```python
from build123d import *

# Parameters (mm, degrees)
SKETCH_W        = 60
SKETCH_H        = 30
SKETCH_R        = 2.25
SKETCH_R_2      = 2.2
PAD_DEPTH       = 2.8
SKETCH001_W     = 75
SKETCH001_H     = 45
POCKET_DEPTH    = 2.801
SKETCH002_R     = 2.2
PAD001_DEPTH    = 24
SKETCH003_R     = 8.1
POCKET001_DEPTH = 3.8
CHAMFER_SIZE    = 2
FILLET_R        = 2
FILLET001_R     = 2


with BuildPart() as part:
    # Sketch → Pad (new body)
    with BuildSketch(Plane.XY):
        Rectangle(SKETCH_W, SKETCH_H)
        with Locations((25, 0)):
            Circle(SKETCH_R, mode=Mode.SUBTRACT)
        with Locations((-25, 0)):
            Circle(SKETCH_R, mode=Mode.SUBTRACT)
        Circle(SKETCH_R_2, mode=Mode.SUBTRACT)
    extrude(amount=PAD_DEPTH)

    # Sketch001 → Pocket (cut, through all)
    with BuildSketch(Plane.XY.offset(2.8)):
        Rectangle(SKETCH001_W, SKETCH001_H)
        with BuildLine():
            ThreePointArc((-27, 9.5), (-24.525126, 10.525126), (-23.5, 13))
            Line((-23.5, 13), (-23.5, 18))
            Line((-23.5, 18), (-3.5, 18))
            Line((-3.5, 18), (-3.5, 13))
            ThreePointArc((-3.5, 13), (0, 9.5), (3.5, 13))
            Line((3.5, 13), (3.5, 18))
            Line((3.5, 18), (23.5, 18))
            Line((23.5, 18), (23.5, 13))
            ThreePointArc((23.5, 13), (24.525126, 10.525126), (27, 9.5))
            Line((27, 9.5), (32, 9.5))
            Line((32, 9.5), (32, -9.5))
            Line((32, -9.5), (27, -9.5))
            ThreePointArc((27, -9.5), (24.525128, -10.525124), (23.5, -12.999994))
            Line((23.5, -12.999994), (23.5, -17.999994))
            Line((23.5, -17.999994), (3.5, -17.999994))
            Line((3.5, -12.999994), (3.5, -17.999994))
            ThreePointArc((3.5, -12.999994), (-4e-06, -9.5), (-3.5, -13.000002))
            Line((-3.5, -13.000002), (-3.5, -18.000002))
            Line((-23.499999, -18.000002), (-3.5, -18.000002))
            Line((-23.499999, -18.000002), (-23.499999, -13.000002))
            ThreePointArc((-23.499999, -13.000002), (-24.525131, -10.525138), (-27, -9.500018))
            Line((-27, -9.500018), (-32, -9.500018))
            Line((-32, -9.500018), (-32, 9.5))
            Line((-32, 9.5), (-27, 9.5))
        make_face(mode=Mode.SUBTRACT)
    extrude(amount=-POCKET_DEPTH, mode=Mode.SUBTRACT)

    # Sketch002 → Pad001 (new body)
    with BuildSketch(Plane.XY.offset(2.8)):
        with BuildLine():
            Line((-10, -10), (-10, 10))
            Line((-10, 10), (-1.802776, 10))
            ThreePointArc((-1.802776, 10), (0, 9.5), (1.802776, 10))
            Line((1.802776, 10), (10, 10))
            Line((10, 10), (10, -10))
            Line((1.802776, -10), (10, -10))
            ThreePointArc((1.802776, -10), (0, -9.5), (-1.802776, -10))
            Line((-1.802776, -10), (-10, -10))
        make_face()
        Circle(SKETCH002_R, mode=Mode.SUBTRACT)
    extrude(amount=PAD001_DEPTH)

    # Sketch003 → Pocket001 (cut)
    with BuildSketch(Plane.XY.offset(26.8)):
        Circle(SKETCH003_R)
    extrude(amount=-POCKET001_DEPTH, mode=Mode.SUBTRACT)

    # Chamfer
    chamfer_edges = [part.edges().sort_by_distance(p)[0] for p in [
        (-10, -10, 14.8),
        (10, -10, 14.8),
        (-10, 10, 14.8),
        (10, 10, 14.8),
    ]]
    chamfer(chamfer_edges, length=CHAMFER_SIZE)

    # Fillet
    fillet_edges = [part.edges().sort_by_distance(p)[0] for p in [
        (-10, 0, 2.8),
    ]]
    fillet(fillet_edges, radius=FILLET_R)

    # Fillet001
    fillet001_edges = [part.edges().sort_by_distance(p)[0] for p in [
        (10, 0, 2.8),
    ]]
    fillet(fillet001_edges, radius=FILLET001_R)


solid = part.part
```
Verification items for the finished model (mm, model axes). A direction names the side the tool comes from. Give positions to 0.01 mm unless a question says otherwise; leave off trailing zeros. Order: outer loops, then holes, each group sorted by start corner. A loop starts at its lowest first (then second) coordinate and runs counter-clockwise, first axis right, second up. Notation, with made-up numbers: M 8,75.5 L 62,75.5 A15 ccw 62,96.5 Z; hole C -11.75,76.5 d5. An arc over 180 degrees is marked long. Answer in a Markdown table with one row per item. Add a question column.
Item 1: Section check B-B, the plane y = 0. Enter the section's corners in (x, z), and give its area (3 significant figures).
Item 2: Tool access check on faces 4 (the flat face through (-28, -9.5, 1)), 5 (the flat face through (-29, 9.5, 1)), 6 (the flat face through (29, -9.5, 1)). Record the directions out of +Z, -Z, +X, -X, +Y, -Y that give a thin tool (end or side, any length) a straight path to the whole face; none if there is none.
Item 3: Section check D-D, the plane x = 9. Enter the section's corners in (y, z), and give its area (3 significant figures).
Item 4: Scan lines: probe 1 along Y at (x, z) = (0, 15); probe 2 along Y at (x, z) = (0, 24); probe 3 along Z at (x, y) = (14.5, -10). Record each from-to range of solid material in increasing order. Write a range as from..to.
Item 5: Section check C-C, the plane z = 15. Enter the section's corners in (x, y), and give its area (3 significant figures).
Item 6: Section check A-A, the plane x = 0. Enter the section's corners in (y, z).
Item 7: Gauge pin test, flat ends, axial feed: pin 1 (1 mm diameter, centred on y = 13.5, z = 1.5, fed in from -X); pin 2 (18 mm diameter, centred on x = 2.5, y = -1, fed in from +Z); pin 3 (7 mm diameter, centred on x = -6, z = 12.5, fed in from -Y); pin 4 (1.4 mm diameter, centred on x = -28, z = 1, fed in from -Y). Record the tip position at first contact, or that the pin passes through.
Item 8: Mould release check, pull along Y, two halves, no side actions. Record for faces 1 (the cylindrical face through (27.146, 0.676, 1.38)), 2 (the flat face through (-23.5, -14, 1)), 3 (the flat face through (-5, 10, 15)): released by +Y, released by -Y, zero draft, split by the parting line, or undercut.
Filled sheet:
| question | item | result |
|---|---|---|
| 1 | outline | M -30,0 L -27.25,0 L -27.25,2.8 L -30,2.8 Z; M -22.75,0 L -2.2,0 L -2.2,23 L -8.1,23 L -8.1,26.8 L -10,26.8 L -10,4.8 A2 cw -12,2.8 L -22.75,2.8 Z; M 2.2,0 L 22.75,0 L 22.75,2.8 L 12,2.8 A2 cw 10,4.8 L 10,26.8 L 8.1,26.8 L 8.1,23 L 2.2,23 Z; M 27.25,0 L 30,0 L 30,2.8 L 27.25,2.8 Z |
| 1 | area | 462 mm^2 |
| 2 | face 4 | +Z, -Z, -X, -Y |
| 2 | face 5 | +Z, -Z, -X, +Y |
| 2 | face 6 | +Z, -Z, +X, -Y |
| 3 | outline | M -15,0 L 15,0 L 15,2.8 L 9,2.8 L 9,26.8 L -9,26.8 L -9,2.8 L -15,2.8 Z |
| 3 | area | 516 mm^2 |
| 4 | probe 1 | y = -9.5..-2.2, 2.2..9.5 |
| 4 | probe 2 | y = -9.5..-8.1, 8.1..9.5 |
| 4 | probe 3 | z = 0..2.8 |
| 5 | outline | M -10,-8 L -8,-10 L -1.8,-10 A3.5 cw 1.8,-10 L 8,-10 L 10,-8 L 10,8 L 8,10 L 1.8,10 A3.5 cw -1.8,10 L -8,10 L -10,8 Z; hole C 0,0 d4.4 |
| 5 | area | 374 mm^2 |
| 6 | outline | M -9.5,0 L -2.2,0 L -2.2,23 L -8.1,23 L -8.1,26.8 L -9.5,26.8 Z; M 2.2,0 L 9.5,0 L 9.5,26.8 L 8.1,26.8 L 8.1,23 L 2.2,23 Z |
| 7 | pin 1 | stops at x = -23.5 |
| 7 | pin 2 | stops at z = 26.8 |
| 7 | pin 3 | stops at y = -10 |
| 7 | pin 4 | stops at y = -9.5 |
| 8 | face 1 | undercut |
| 8 | face 2 | zero draft |
| 8 | face 3 | released by +Y |
